Geometry: final body of the model. Coordinates: model frame, mm. A direction names the side the tool comes from. Give positions to 0.01 mm unless a question says otherwise; leave off trailing zeros. Write each loop counter-clockwise with the first axis right and the second up, starting at its lowest first coordinate (ties: lowest second). Pieces come first, ordered by that corner, then holes.
from build123d import *

# Parameters (mm, degrees)
EXTRUDE_1_DEPTH = 4
SKETCH_3_R      = 7.5
EXTRUDE_2_DEPTH = 6.5


with BuildPart() as part:
    # 草图1 → 凸台-拉伸1 (new body)
    with BuildSketch(Plane.XY):
        with BuildLine():
            Line((-10, -20), (10, -20))
            ThreePointArc((10, -20), (24.142135624, -14.142135624), (30, 0))
            Line((30, 0), (30, 10))
            ThreePointArc((30, 10), (27.071067812, 17.071067812), (20, 20))
            Line((20, 20), (11.249888888, 20))
            ThreePointArc((11.249888888, 20), (0, 14.4), (-11.249888888, 20))
            Line((-11.249888888, 20), (-20, 20))
            ThreePointArc((-20, 20), (-27.071067812, 17.071067812), (-30, 10))
            Line((-30, 10), (-30, 0))
            ThreePointArc((-30, 0), (-24.142135624, -14.142135624), (-10, -20))
        make_face()
    extrude(amount=EXTRUDE_1_DEPTH)

    # 草图3 → 凸台-拉伸2 (add)
    with BuildSketch(Plane.XY):
        with Locations((-12.5, 0)):
            Circle(SKETCH_3_R)
        with Locations((12.5, 0)):
            Circle(SKETCH_3_R)
    extrude(amount=-EXTRUDE_2_DEPTH)


solid = part.part
Q1. Section C-C on x = -12.5. Output: boundary loops of the cut face in (y, z), plus the area to 3 significant figures.
Filled sheet:
outline: (-19.84, 0) - (-7.5, 0) - (-7.5, -6.5) - (7.5, -6.5) - (7.5, 0) - (20, 0) - (20, 4) - (-19.84, 4) - close
area: 257 mm2
Q2. Section D-D on z = -4. Output: boundary loops of the cut face in (x, y).
Filled sheet:
outline: circle Ø15 at (-12.5, 0); circle Ø15 at (12.5, 0)
Q3. Section A-A on z = 2. Output: boundary loops of the cut face in (x, y), plus the area to 3 significant figures.
Filled sheet:
outline: (-30, 0) arc R20 ccw to (-10, -20) - (10, -20) arc R20 ccw to (30, 0) - (30, 10) arc R10 ccw to (20, 20) - (11.25, 20) arc R14.1 cw to (-11.25, 20) - (-20, 20) arc R10 ccw to (-30, 10) - close
area: 2,100 mm2
Q4. Pull-direction query (X, two-part tool) for faces 3 (the cylindrical face through (-26.99, 17.15, 1.97)), 4 (the cylindrical face through (0.2, 14.4, 2)), 5 (the flat face through (-13, 0, -6.5)); classes: released by +X, released by -X, zero draft, split by the parting line, or undercut.
Filled sheet:
face 3: released by -X
face 4: undercut
face 5: zero draft
Q5. Pin query (flat end, axial travel): P1, Ø4, axis at x = -5, y = 10.5, coming from the -Z side; P2, Ø4, axis at y = 11, z = -4, coming from the -X side. Return the tip coordinate at first contact, or that it passes through.
Filled sheet:
P1: stops at z = 0
P2: passes through
Q6. Ray query, line 1 along Z through (x, y) = (21, 11); line 2 along X through (y, z) = (3, -6); line 3 along X through (y, z) = (4.5, -3). Return the intervals inside material, ascending.
Filled sheet:
line 1: z = 0 to 4
line 2: x = -19.37 to -5.63, 5.63 to 19.37
line 3: x = -18.5 to -6.5, 6.5 to 18.5
Q7. Access query for faces 1 (the cylindrical face through (-20, 0, -3)), 2 (the flat face through (-30, 5, 2)). Directions: +Z, -Z, +X, -X, +Y, -Y. A direction counts if a zero-diameter tool reaches every point of the face in a straight line with its end or side. Return the directions, or none.
Filled sheet:
face 1: -Z
face 2: +Z, -Z, -X, +Y, -Y
Q8. Section B-B on y = -3.5. Output: boundary loops of the cut face in (x, z).
Filled sheet:
outline: (-29.69, 0) - (-19.13, 0) - (-19.13, -6.5) - (-5.87, -6.5) - (-5.87, 0) - (5.87, 0) - (5.87, -6.5) - (19.13, -6.5) - (19.13, 0) - (29.69, 0) - (29.69, 4) - (-29.69, 4) - close
